```python
from build123d import *

# Parameters (mm, degrees)
SKETCH1_W             = 10
SKETCH1_H             = 10
BOSS_EXTRUDE1_DEPTH   = 80
BOSS_EXTRUDE1_2_DEPTH = 80
BOSS_EXTRUDE1_3_DEPTH = 80
BOSS_EXTRUDE1_4_DEPTH = 80
SKETCH2_W             = 140
SKETCH2_H             = 120
BOSS_EXTRUDE2_DEPTH   = 10
FILLET1_R             = 10


with BuildPart() as part:
    # Sketch1 → Boss-Extrude1 (new body)
    with BuildSketch(Plane(origin=(0, 0, 0), x_dir=(1, 0, 0), z_dir=(0, 1, 0))):
        with Locations((-5, 95)):
            Rectangle(SKETCH1_W, SKETCH1_H)
    extrude(amount=BOSS_EXTRUDE1_DEPTH)



with BuildPart() as body_2:
    # Sketch1 → Boss-Extrude1 2 (new body)
    with BuildSketch(Plane(origin=(0, 0, 0), x_dir=(1, 0, 0), z_dir=(0, 1, 0))):
        with Locations((-5, 5)):
            Rectangle(SKETCH1_W, SKETCH1_H)
    extrude(amount=BOSS_EXTRUDE1_2_DEPTH)


with BuildPart() as body_3:
    # Sketch1 → Boss-Extrude1 3 (new body)
    with BuildSketch(Plane(origin=(0, 0, 0), x_dir=(1, 0, 0), z_dir=(0, 1, 0))):
        with Locations((-95, 5)):
            Rectangle(SKETCH1_W, SKETCH1_H)
    extrude(amount=BOSS_EXTRUDE1_3_DEPTH)


with BuildPart() as body_4:
    # Sketch1 → Boss-Extrude1 4 (new body)
    with BuildSketch(Plane(origin=(0, 0, 0), x_dir=(1, 0, 0), z_dir=(0, 1, 0))):
        with Locations((-95, 95)):
            Rectangle(SKETCH1_W, SKETCH1_H)
    extrude(amount=BOSS_EXTRUDE1_4_DEPTH)


with BuildPart() as part_1:
    add(part.part)

    add(body_2.part)  # Boss-Extrude2 merges body 2

    add(body_3.part)  # Boss-Extrude2 merges body 3

    add(body_4.part)  # Boss-Extrude2 merges body 4
    # Sketch2 → Boss-Extrude2 (add)
    with BuildSketch(Plane(origin=(0, 80, 0), x_dir=(1, 0, 0), z_dir=(0, 1, 0))):
        with Locations((-50, 50)):
            Rectangle(SKETCH2_W, SKETCH2_H)
    extrude(amount=BOSS_EXTRUDE2_DEPTH)

    # Fillet1
    fillet1_edges = [part_1.edges().sort_by_distance(p)[0] for p in [
        (-120, 85, -110),
        (-120, 85, 10),
        (20, 85, 10),
        (20, 85, -110),
    ]]
    fillet(fillet1_edges, radius=FILLET1_R)


solid = part_1.part
```
CAD build for the part. Positions are in the model's coordinates, mm. A direction names the side the tool comes from. Round coordinates to 2 decimals unless told otherwise and drop trailing zeros. Loops run counter-clockwise (first coordinate to the right, second up) from the corner with the lowest first, then second, coordinate; pieces in that order, holes last. Notation, with made-up numbers: M 38.5,-11 L 81.5,-11 A9 ccw 81.5,0 Z; hole C -37,12 d9. An arc over 180 degrees is marked long. Use a Markdown table: item, result. Add a question column.
(1) Cut at B-B (x = -97). Give the cut face in (y, z).
(2) Cut at C-C (z = -42). Give the cut face in (x, y).
(3) Cut at A-A (y = 62.5). Give the cut face in (x, z).
(4) Which spindle directions (+Z, -Z, +X, -X, +Y, -Y) get a long thin tool onto all of the face, cutting with end or side? Do faces 4 (the face through (-95, 39, 0)), 5 (the face through (-10, 39, -95)), 6 (the face through (-95, 39, -100)), 7 (the face through (-5, 39, -90)). Say none if no direction does.
(5) Flat gauge pins, fed straight in: pin 1 (8 mm diameter, centred on x = -95.5, y = 57, fed in from +Z); pin 2 (8 mm diameter, centred on y = 54.5, z = -7, fed in from -X); pin 3 (11 mm diameter, centred on y = 25, z = -94.5, fed in from +X); pin 4 (3 mm diameter, centred on x = -12, y = 26, fed in from -Z). Where does each tip first touch, or does it go through?
(6) Drill centre lines: line 1 (X direction, y = 25.5, z = -3.5); line 2 (Y direction, x = -99, z = -31). Where is each one in solid material? Low to high.
(7) Cut at D-D (x = -46). Give the cut face in (y, z), and give its area (3 significant figures).
(8) Pull direction Z, two halves, no side cores. Call faces 1 (the face through (-95, 0, -95)), 2 (the face through (-5, 39, 0)), 3 (the face through (-95, 39, -10)): +Z half, -Z half, draft (parallel to the pull), parting line (faces both ways), or undercut.
Geometry says:
| question | item | result |
|---|---|---|
| 1 | outline | M 0,-100 L 80,-100 L 80,-110 L 90,-110 L 90,10 L 80,10 L 80,0 L 0,0 L 0,-10 L 80,-10 L 80,-90 L 0,-90 Z |
| 2 | outline | M -120,80 L 20,80 L 20,90 L -120,90 Z |
| 3 | outline | M -100,-100 L -90,-100 L -90,-90 L -100,-90 Z; M -100,-10 L -90,-10 L -90,0 L -100,0 Z; M -10,-100 L 0,-100 L 0,-90 L -10,-90 Z; M -10,-10 L 0,-10 L 0,0 L -10,0 Z |
| 4 | face 4 | +Z, +X, -X, -Y |
| 4 | face 5 | +Z, -Z, -Y |
| 4 | face 6 | -Z, +X, -X, -Y |
| 4 | face 7 | +X, -X, -Y |
| 5 | pin 1 | stops at z = 0 |
| 5 | pin 2 | stops at x = -100 |
| 5 | pin 3 | stops at x = 0 |
| 5 | pin 4 | passes through |
| 6 | line 1 | x = -100 to -90, -10 to 0 |
| 6 | line 2 | y = 80 to 90 |
| 7 | outline | M 80,-110 L 90,-110 L 90,10 L 80,10 Z |
| 7 | area | 1,200 mm² |
| 8 | face 1 | draft |
| 8 | face 2 | +Z half |
| 8 | face 3 | undercut |
